from build123d import *

# Parameters (mm, degrees)
F3_R     = 4.5
F4_DEPTH = 25
F5_W     = 17
F5_H     = 14
F6_DEPTH = 25
F8_DEPTH = 25
F9_SIZE  = 1
F10_R    = 1


with BuildPart() as f2:
    # F0 (on Front) → F2 (revolve)
    with BuildSketch(Plane.XZ):
        Polygon((0, 45), (0, 10), (28, 10), (28, 22.5), (12, 22.5), (12, 45), align=None)
    revolve(axis=Axis((18.0693501607, 0, 0), (1, 0, 0)))

    # F3 (on Top) → F4 (cut, symmetric)
    with BuildSketch(Plane.XY):
        with Locations((20, 0)):
            Circle(F3_R)
    extrude(amount=F4_DEPTH, both=True, mode=Mode.SUBTRACT)

    # F5 (on face) → F6 (cut)
    with BuildSketch(Plane.YZ.offset(12)):
        with Locations((0, 43)):
            Rectangle(F5_W, F5_H)
    extrude(amount=-F6_DEPTH, mode=Mode.SUBTRACT)

    # F7 (on Right) → F8 (cut)
    with BuildSketch(Plane.YZ):
        Polygon((26.9269145362, 25.3612159322), (31.1769145362, 18), (40.5253827808, 23.3973406575), (36.2753827808, 30.7585565897), align=None)
        Polygon((40.5253827808, 23.3973406575), (31.1769145362, 18), (35.4269145362, 10.6387840678), (44.7753827808, 16.0361247254), align=None)
    extrude(amount=F8_DEPTH, mode=Mode.SUBTRACT)

    # F9
    f9_edges = [f2.edges().sort_by_distance(p)[0] for p in [
        (28, 0, -22.5),
        (12, 22.5, 38.971143),
        (0, 22.5, 38.971143),
        (0, -22.5, -38.971143),
        (12, -22.5, -38.971143),
    ]]
    chamfer(f9_edges, length=F9_SIZE)

    # F10
    f10_edges = [f2.edges().sort_by_distance(p)[0] for p in [
        (12, 0, -22.5),
    ]]
    fillet(f10_edges, radius=F10_R)


solid = f2.part
Input: part model. Units: mm. Frame: model coordinates. A direction names the side the tool comes from. Give positions to 0.01 mm unless a question says otherwise; leave off trailing zeros. Order: outer loops, then holes, each group sorted by start corner. A loop starts at its lowest first (then second) coordinate and runs counter-clockwise, first axis right, second up. Notation, with made-up numbers: (42, 48.5) -> (56, 48.5) arc R15 ccw to (56, 53.5) -> close; hole circle Ø11 at (23, -31). An arc over 180 degrees is marked (long way). Use one line per item in the form item = value.
1) Reachability of faces 4 (the flat face through (5.92, 31.12, 18.1)), 5 (the flat face through (5.916, 30.523, 27.437)), 6 (the flat face through (5.916, 38.924, 12.658)) from +Z, -Z, +X, -X, +Y, -Y: full face, straight path, thin tool, end or side. Return the list, or none.
Response values:
face_4 = +X, -X
face_5 = +X, -X, +Y
face_6 = +Z, +X, -X
2) Section A-A, the plane y = 0. Return loops of the section in (x, z).
Response values:
outline = (0, -44) -> (1, -45) -> (11, -45) -> (12, -44) -> (12, -23.5) arc R1 cw to (13, -22.5) -> (15.5, -22.5) -> (15.5, -10) -> (0, -10) -> close; (0, 10) -> (15.5, 10) -> (15.5, 22.5) -> (13, 22.5) arc R1 cw to (12, 23.5) -> (12, 36) -> (0, 36) -> close; (24.5, -22.5) -> (27, -22.5) -> (28, -21.5) -> (28, -10) -> (24.5, -10) -> close; (24.5, 10) -> (28, 10) -> (28, 21.5) -> (27, 22.5) -> (24.5, 22.5) -> close
3) Mould query, pull axis Y, two halves, no side actions, for faces 1 (the flat face through (6, 8.5, 40)), 2 (the flat face through (12, 19, -19)), 3 (the conical face through (11.84, 22.26, 38.14)). Classes: pulls with the +Y half, pulls with the -Y half, needs draft (parallel to the pull), parting line crosses it, or undercut.
Response values:
face_1 = undercut
face_2 = needs draft
face_3 = pulls with the +Y half
4) Section D-D, the plane x = 4.5. Return loops of the section in (y, z), and give its area (3 significant figures).
Response values:
outline = (-8.5, 36) -> (-8.5, 44.19) arc R45 ccw (long way) to (42.52, 14.73) -> (35.43, 10.64) -> (26.93, 25.36) -> (34.02, 29.46) arc R45 ccw to (8.5, 44.19) -> (8.5, 36) -> close; hole circle Ø20 at (0, 0)
area = 5,750 mm^2
5) Section C-C, the plane x = 22.25. Return loops of the section in (y, z).
Response values:
outline = (-3.9, -22.16) -> (-3.9, -9.21) arc R10 cw to (-3.9, 9.21) -> (-3.9, 22.16) arc R22.5 ccw to start; (3.9, -22.16) arc R22.5 ccw to (3.9, 22.16) -> (3.9, 9.21) arc R10 cw to (3.9, -9.21) -> close
6) First-contact query: pin 1 Ø8 at (y, z) = (-3, -1.5) entering from +X; pin 2 Ø5 at (x, y) = (9, -18) entering from +Z; pin 3 Ø1 at (x, z) = (5.5, 25.5) entering from +Y; pin 4 Ø10 at (x, y) = (3.5, 16.5) entering from +Z. Flat tips, straight axial feed; report the tip coordinate or a pass-through.
Response values:
pin_1 = through
pin_2 = 42.25
pin_3 = 28.03
pin_4 = 43.51
7) Line query: probe 1 along X at (y, z) = (0, 19.25); probe 2 along Y at (x, z) = (6.75, -7); probe 3 along Y at (x, z) = (20, -17.5). Output: solid intervals per line, ascending.
Response values:
probe_1 = 0 to 15.5, 24.5 to 28
probe_2 = -44.45 to -7.14, 7.14 to 44.45
probe_3 = -14.14 to -4.5, 4.5 to 14.14
8) Section B-B, the plane z = 0. Return loops of the section in (x, y), and give its area (3 significant figures).
Response values:
outline = (0, -44) -> (1, -45) -> (11, -45) -> (12, -44) -> (12, -23.5) arc R1 cw to (13, -22.5) -> (27, -22.5) -> (28, -21.5) -> (28, -10) -> (0, -10) -> close; (0, 10) -> (28, 10) -> (28, 21.5) -> (27, 22.5) -> (13, 22.5) arc R1 cw to (12, 23.5) -> (12, 44) -> (11, 45) -> (1, 45) -> (0, 44) -> close
area = 1,240 mm^2
